from build123d import *

# Parameters (mm, degrees)
BOSS_EXTRUDE1_DEPTH = 20
SKETCH5_R           = 1.75
CUT_EXTRUDE3_DEPTH  = 45.590264942
SKETCH6_R           = 1.75
CUT_EXTRUDE4_DEPTH  = 45.590264942
CUT_EXTRUDE5_DEPTH  = 45.590264942
CUT_EXTRUDE6_DEPTH  = 45.590264942
BOSS_EXTRUDE3_DEPTH = 10
SKETCH10_R          = 2.85
CUT_EXTRUDE7_DEPTH  = 4.933726003
BOSS_EXTRUDE4_DEPTH = 10
SKETCH12_R          = 2.85
CUT_EXTRUDE8_DEPTH  = 4.933726003
CUT_EXTRUDE9_DEPTH  = 41
CHAMFER1_SIZE       = 1
CHAMFER2_SIZE       = 0.5
FILLET1_R           = 1
FILLET2_R           = 3


with BuildPart() as part:
    # Sketch1 → Boss-Extrude1 (new body)
    with BuildSketch(Plane.XY):
        Polygon((-16.499999997, 0), (-0.605600394, 0), (-0.605600394, 13.845143912), (10.605600394, 13.845143912), (10.605600394, 0), (26.499999997, 0), (29.800788035, 3.933726003), (17.736610648, 14.0567728), (28.429456198, 26.800009899), (24.599233982, 30.013947947), (13.906388432, 17.270710848), (7.395010666, 22.73440553), (18.087856216, 35.47764263), (14.257634, 38.691580678), (5, 27.658762099), (-4.257634, 38.691580678), (-8.087856216, 35.47764263), (2.604989334, 22.73440553), (-3.906388432, 17.270710848), (-14.599233982, 30.013947947), (-18.429456198, 26.800009899), (-7.736610648, 14.0567728), (-19.800788035, 3.933726003), align=None)
    extrude(amount=BOSS_EXTRUDE1_DEPTH)

    # Sketch5 → Cut-Extrude3 (cut, through all)
    with BuildSketch(Plane(origin=(2.381579924, 1.998382835, 0), x_dir=(0, 0, 1), z_dir=(-0.766044443, -0.64278761, 0))):
        with Locations((5.02612125, 26.624225366)):
            Circle(SKETCH5_R)
    extrude(amount=-CUT_EXTRUDE3_DEPTH, mode=Mode.SUBTRACT)

    # Sketch6 → Cut-Extrude4 (cut, through all)
    with BuildSketch(Plane(origin=(3.486660965, -2.92565593, 0), x_dir=(0, 0, -1), z_dir=(0.766044443, -0.64278761, 0))):
        with Locations((-5.02612125, 33.052101463)):
            Circle(SKETCH6_R)
    extrude(amount=-CUT_EXTRUDE4_DEPTH, mode=Mode.SUBTRACT)

    # Sketch7 → Cut-Extrude5 (cut, through all)
    with BuildSketch(Plane(origin=(2.381579924, 1.998382835, 0), x_dir=(0, 0, 1), z_dir=(-0.766044443, -0.64278761, 0))):
        with BuildLine():
            ThreePointArc((0, 25.376224756), (2.050252532, 30.325972224), (7, 32.376224756))
            Line((7, 32.376224756), (0, 32.376224756))
            Line((0, 32.376224756), (0, 25.376224756))
        make_face()
        with BuildLine():
            ThreePointArc((7, 32.376224756), (11.421832756, 31.087378042), (14.458671842, 27.62452674))
            Line((14.458671842, 27.62452674), (20, 15.741110157))
            Line((20, 15.741110157), (20, 32.376224756))
            Line((20, 32.376224756), (7, 32.376224756))
        make_face()
    extrude(amount=-CUT_EXTRUDE5_DEPTH, mode=Mode.SUBTRACT)

    # Sketch8 → Cut-Extrude6 (cut, through all)
    with BuildSketch(Plane(origin=(3.486660965, -2.92565593, 0), x_dir=(0, 0, -1), z_dir=(0.766044443, -0.64278761, 0))):
        with BuildLine():
            Line((-20, 22.168986254), (-14.458671842, 34.052402837))
            ThreePointArc((-14.458671842, 34.052402837), (-11.421832756, 37.515254138), (-7, 38.804100853))
            Line((-7, 38.804100853), (-20, 38.804100853))
            Line((-20, 38.804100853), (-20, 22.168986254))
        make_face()
        with BuildLine():
            Line((0, 38.804100853), (-7, 38.804100853))
            ThreePointArc((-7, 38.804100853), (-2.050252532, 36.753848321), (0, 31.804100853))
            Line((0, 31.804100853), (0, 38.804100853))
        make_face()
    extrude(amount=-CUT_EXTRUDE6_DEPTH, mode=Mode.SUBTRACT)

    # Sketch9 → Boss-Extrude3 (add)
    with BuildSketch(Plane.XY.offset(20)):
        Polygon((-0.605600394, 0), (-16.499999997, 0), (-19.800788035, 3.933726003), (-0.605600394, 3.933726003), align=None)
        Polygon((10.605600394, 3.933726003), (10.605600394, 0), (26.499999997, 0), (29.800788035, 3.933726003), align=None)
    extrude(amount=BOSS_EXTRUDE3_DEPTH)

    # Sketch10 → Cut-Extrude7 (cut, through all)
    with BuildSketch(Plane(origin=(0, 3.933726003, 0), x_dir=(1, 0, 0), z_dir=(0, 1, 0))):
        with Locations((-8.552800195, -25)):
            Circle(SKETCH10_R)
        with Locations((18.552800195, -25)):
            Circle(SKETCH10_R)
    extrude(amount=-CUT_EXTRUDE7_DEPTH, mode=Mode.SUBTRACT)

    # Sketch11 → Boss-Extrude4 (add)
    with BuildSketch(Plane(origin=(0, 0, 0), x_dir=(-1, 0, 0), z_dir=(0, 0, -1))):
        Polygon((19.800788035, 3.933726003), (16.499999997, 0), (0.605600394, 0), (0.605600394, 3.933726003), align=None)
        Polygon((-10.605600394, 3.933726003), (-10.605600394, 0), (-26.499999997, 0), (-29.800788035, 3.933726003), align=None)
    extrude(amount=BOSS_EXTRUDE4_DEPTH)

    # Sketch12 → Cut-Extrude8 (cut, through all)
    with BuildSketch(Plane(origin=(0, 3.933726003, 0), x_dir=(1, 0, 0), z_dir=(0, 1, 0))):
        with Locations((-8.552800195, 5)):
            Circle(SKETCH12_R)
        with Locations((18.552800195, 5)):
            Circle(SKETCH12_R)
    extrude(amount=-CUT_EXTRUDE8_DEPTH, mode=Mode.SUBTRACT)

    # Sketch13 → Cut-Extrude9 (cut, through all)
    with BuildSketch(Plane.XY.offset(30)):
        Polygon((-16.499999997, 0), (-16.499999997, 3.933726003), (-16.499999997, 6.703416029), (-19.800788035, 3.933726003), align=None)
        Polygon((26.499999997, 0), (26.499999997, 3.933726003), (26.499999997, 6.703416029), (29.800788035, 3.933726003), align=None)
    extrude(amount=-CUT_EXTRUDE9_DEPTH, mode=Mode.SUBTRACT)

    # Chamfer1
    chamfer1_edges = [part.edges().sort_by_distance(p)[0] for p in [
        (-0.560320061, 34.285293508, 3.27612125),
        (-14.732142259, 22.393722729, 3.27612125),
        (10.560320061, 34.285293508, 6.77612125),
        (24.732142259, 22.393722729, 6.77612125),
    ]]
    chamfer(chamfer1_edges, length=CHAMFER1_SIZE)

    # Chamfer2
    chamfer2_edges = [part.edges().sort_by_distance(p)[0] for p in [
        (-11.402800195, 3.933726003, 25),
        (15.702800195, 3.933726003, 25),
        (15.702800195, 3.933726003, -5),
        (-11.402800195, 3.933726003, -5),
    ]]
    chamfer(chamfer2_edges, length=CHAMFER2_SIZE)

    # Fillet1
    fillet1_edges = [part.edges().sort_by_distance(p)[0] for p in [
        (-0.605600394, 8.889434958, 20),
        (10.605600394, 8.889434958, 20),
        (-8.552800195, 3.933726003, 20),
        (-0.605600394, 3.933726003, 25),
        (-0.605600394, 1.966863002, 30),
        (-8.552800195, 3.933726003, 30),
        (10.605600394, 3.933726003, 25),
        (10.605600394, 1.966863002, 30),
        (10.605600394, 8.889434958, 0),
        (-0.605600394, 8.889434958, 0),
        (-0.605600394, 3.933726003, -5),
        (-0.605600394, 1.966863002, -10),
        (18.552800195, 3.933726003, 0),
        (10.605600394, 3.933726003, -5),
        (18.552800195, 3.933726003, -10),
        (10.605600394, 1.966863002, -10),
        (26.499999997, 1.966863002, -10),
        (-8.552800195, 3.933726003, -10),
        (-8.552800195, 3.933726003, 0),
        (18.552800195, 3.933726003, 30),
        (18.552800195, 3.933726003, 20),
        (26.499999997, 1.966863002, 30),
        (26.499999997, 5.318571016, 20),
        (26.499999997, 5.318571016, 0),
        (26.499999997, 3.933726003, -5),
        (26.499999997, 3.933726003, 25),
        (-16.499999997, 1.966863002, 30),
        (-16.499999997, 5.318571016, 20),
        (-16.499999997, 3.933726003, 25),
        (-16.499999997, 1.966863002, -10),
        (-16.499999997, 3.933726003, -5),
        (-16.499999997, 5.318571016, 0),
    ]]
    fillet(fillet1_edges, radius=FILLET1_R)

    # Fillet2
    fillet2_edges = [part.edges().sort_by_distance(p)[0] for p in [
        (5, 27.658762099, 9.479415808),
        (-7.736610648, 14.0567728, 10),
        (-3.906388432, 17.270710848, 10),
        (2.604989334, 22.73440553, 10),
        (7.395010666, 22.73440553, 10),
        (13.906388432, 17.270710848, 10),
        (17.736610648, 14.0567728, 10),
    ]]
    fillet(fillet2_edges, radius=FILLET2_R)


solid = part.part
Part model, mm, in its own coordinate system. A direction names the side the tool comes from. Round coordinates to 2 decimals unless told otherwise and drop trailing zeros. Write each loop counter-clockwise with the first axis right and the second up, starting at its lowest first coordinate (ties: lowest second). Pieces come first, ordered by that corner, then holes. Notation, with made-up numbers: M 65,-30.5 L 97,-30.5 A16 cw 97,-16.5 Z; hole C -30,-17 d4. An arc over 180 degrees is marked long. Return JSON: item names as keys, results as strings. Group by question number.
(1) Saw through at C-C on x = -6.5. Count the separate pieces of the cut face and the enclosed holes in it, then the cut area to 3 significant figures.
(2) Saw through at A-A on z = 25. Write the cut outline in (x, y), then the cut area to 3 significant figures.
(3) Two-plate mould, pull along X, no slides. Class faces 5 (the face through (22.02, 23.79, 3.41)), 6 (the face through (23.31, 9.38, 9.86)), 7 (the face through (-9, 0, 10)): +X half, -X half, draft (parallel to the pull), parting line (faces both ways), or undercut.
(4) Drill centre lines: probe 1 along X at (y, z) = (1, -5); probe 2 along X at (y, z) = (22, 8); probe 3 along X at (y, z) = (19, 1.5). Where is each one in solid material? Low to high.
(5) Pin check, flat tips, straight feed: pin 1 Ø9 at (x, z) = (-11.5, -5) entering from +Y; pin 2 Ø7 at (y, z) = (4, 19) entering from -X; pin 3 Ø4 at (x, y) = (-11.5, 16) entering from +Z; pin 4 Ø5 at (x, z) = (-8.55, 25) entering from -Y. Stop position of each tip, or through.
(6) Which spindle directions (+Z, -Z, +X, -X, +Y, -Y) get a long thin tool onto all of the face, cutting with end or side? Do faces 1 (the face through (-16.5, 3, 10)), 2 (the face through (-0.606, 5, 10)), 3 (the face through (8.63, 22.88, 10.14)), 4 (the face through (18.7, 3.934, -8.5)). Say none if no direction does.
Returned:
{
 "1": {"separate pieces": "4", "enclosed holes": "0", "area": "474 mm²"},
 "2": {"outline": "M -16.5,0 L -11.4,0 L -11.4,3.43 L -11.9,3.93 L -15.5,3.93 A1 ccw -16.5,2.93 Z; M -5.7,0 L -0.61,0 L -0.61,2.93 A1 ccw -1.61,3.93 L -5.2,3.93 L -5.7,3.43 Z; M 10.61,0 L 15.7,0 L 15.7,3.43 L 15.2,3.93 L 11.61,3.93 A1 ccw 10.61,2.93 Z; M 21.4,0 L 26.5,0 L 26.5,2.93 A1 ccw 25.5,3.93 L 21.9,3.93 L 21.4,3.43 Z", "area": "78.8 mm²"},
 "3": {"face 5": "undercut", "face 6": "+X half", "face 7": "draft"},
 "4": {"probe 1": "-16.5 to -11.4, -5.7 to -0.61, 10.61 to 15.7, 21.4 to 26.5", "probe 2": "-14.4 to -7.87, 1.17 to 8.83, 17.87 to 24.4", "probe 3": "-11.88 to -5.2, -1.87 to 11.87, 15.2 to 21.88"},
 "5": {"pin 1": "y = 4.07", "pin 2": "x = -16.5", "pin 3": "z = 18.72", "pin 4": "through"},
 "6": {"face 1": "+Z, -Z, -X, -Y", "face 2": "+Z, -Z, -Y", "face 3": "+Z, -Z", "face 4": "-Z, +X, -X, +Y"}
}
